Answer from the drawing. Dimensions are ordinates in mm from the lowest x, y and z of the part. Round coordinates to 2 decimals unless told otherwise and drop trailing zeros. Order: outer loops, then holes, each group sorted by start corner. A loop starts at its lowest first (then second) coordinate and runs counter-clockwise, first axis right, second up. Notation, with made-up numbers: (76.25, -33) -> (111.25, -33) arc R20 cw to (111.25, 5) -> close; hole circle Ø1 at (21, 12). An arc over 180 degrees is marked (long way). Use a Markdown table: item, result. Add a question column.
Item 1: A flat-ended cylindrical pin translates along its axis: P1, Ø0.8, axis at x = 4, z = 1, coming from the -Y side. Find the tip coordinate at first contact, or state that the pin passes through.
Item 2: Find the intervals of material crossed by L1, parallel to X at y = 8.5, z = 0.9; L2, parallel to Y at x = 62.5, z = 0.75; L3, parallel to Y at x = 9, z = 2.1, in increasing order. Write a range as [from, to].
Item 3: A cutting plane is placed at B-B, the plane z = 0.8. Determine the outline of the cut face in (x, y).
Item 4: A cutting plane is placed at C-C, the plane x = 56.5. Determine the outline of the cut face in (y, z).
Item 5: A cutting plane is placed at A-A, the plane y = 10. Determine the outline of the cut face in (x, z), plus the area to 3 significant figures.
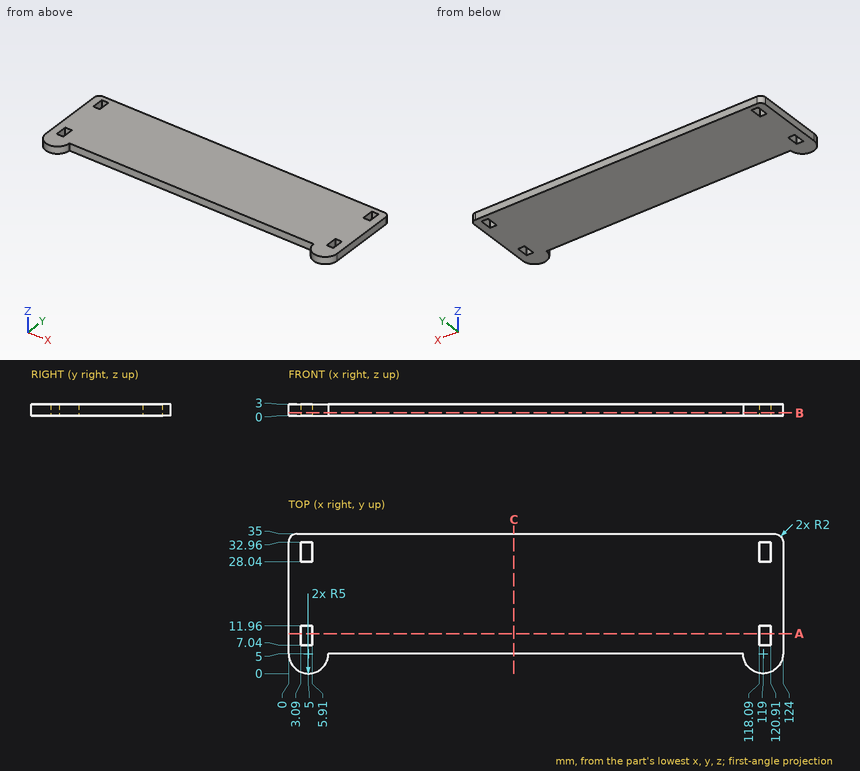
Reported:
| question | item | result |
|---|---|---|
| 1 | P1 | y = 0.04 |
| 2 | L1 | [0, 3.09], [5.91, 118.09], [120.91, 124] |
| 2 | L2 | [5, 35] |
| 2 | L3 | [2, 35] |
| 3 | outline | (0, 5) arc R5 ccw to (10, 5) -> (114, 5) arc R5 ccw to (124, 5) -> (124, 33) arc R2 ccw to (122, 35) -> (2, 35) arc R2 ccw to (0, 33) -> close; hole (3.09, 7.04) -> (5.91, 7.04) -> (5.91, 11.96) -> (3.09, 11.96) -> close; hole (3.09, 28.04) -> (5.91, 28.04) -> (5.91, 32.96) -> (3.09, 32.96) -> close; hole (118.09, 7.04) -> (120.91, 7.04) -> (120.91, 11.96) -> (118.09, 11.96) -> close; hole (118.09, 28.04) -> (120.91, 28.04) -> (120.91, 32.96) -> (118.09, 32.96) -> close |
| 4 | outline | (5, 0) -> (35, 0) -> (35, 3) -> (5, 3) -> close |
| 5 | outline | (0, 0) -> (3.09, 0) -> (3.09, 3) -> (0, 3) -> close; (5.91, 0) -> (118.09, 0) -> (118.09, 3) -> (5.91, 3) -> close; (120.91, 0) -> (124, 0) -> (124, 3) -> (120.91, 3) -> close |
| 5 | area | 355 mm² |
